```python
from build123d import *

# Parameters (mm, degrees)
BOSS_EXTRUDE1_DEPTH     = 100
BOSS_EXTRUDE2_DEPTH     = 100
CUT_EXTRUDE1_DEPTH      = 10
CHAMFER1_SIZE           = 5.5
CHAMFER2_SIZE           = 4
SKETCH8_R               = 2
BOSS_EXTRUDE3_DEPTH     = 9.3
CUT_EXTRUDE3_DEPTH      = 125.214315536
CUT_EXTRUDE3_DEPTH_BACK = 10
SKETCH9_W               = 11
SKETCH9_H               = 9.3
CHAMFER3_SIZE           = 4
CHAMFER4_SIZE           = 3
CHAMFER5_SIZE           = 3
SKETCH10_W              = 5
SKETCH10_H              = 10
CUT_EXTRUDE4_DEPTH      = 94
CHAMFER7_SIZE           = 1
CHAMFER8_SIZE           = 1
SKETCH11_R              = 2.05
CUT_EXTRUDE5_DEPTH      = 10
CHAMFER9_SIZE           = 0.5
SKETCH12_R              = 2
CUT_EXTRUDE6_DEPTH      = 30
BOSS_EXTRUDE6_START     = -2
BOSS_EXTRUDE6_DEPTH     = 10
SKETCH17_R              = 2
CUT_EXTRUDE7_DEPTH      = 17.1
SKETCH19_W              = 50
SKETCH19_H              = 7
CUT_EXTRUDE13_DEPTH     = 17.1
SKETCH20_W              = 62.3
SKETCH20_H              = 63.674798271
CUT_EXTRUDE14_DEPTH     = 15
CHAMFER10_SIZE          = 5
CHAMFER11_SIZE          = 2


with BuildPart() as part:
    # Sketch4 → Boss-Extrude1 (new body)
    with BuildSketch(Plane.XY):
        Polygon((-18.358738987, 4.974798271), (-27, 4.974798271), (-27, -6.2), (27, -6.2), (27, 4.974798271), (18.358738987, 4.974798271), (21.346410162, -0.2), (-21.346410162, -0.2), align=None)
    extrude(amount=BOSS_EXTRUDE1_DEPTH)

    # Sketch6 → Boss-Extrude2 (add)
    with BuildSketch(Plane.XY.offset(100)):
        Polygon((-24.15, 4.974798271), (-24.15, 52.474798271), (-5.5, 52.474798271), (-5.5, 57.474798271), (-31.15, 57.474798271), (-31.15, -6.2), (-24.15, -6.2), align=None)
        Polygon((24.15, -6.2), (24.15, 52.474798271), (5.5, 52.474798271), (5.5, 57.474798271), (31.15, 57.474798271), (31.15, -6.2), align=None)
    extrude(amount=-BOSS_EXTRUDE2_DEPTH)

    # Sketch7 → Cut-Extrude1 (cut)
    with BuildSketch(Plane(origin=(31.15, 0, 0), x_dir=(0, 0, -1), z_dir=(1, 0, 0))):
        Polygon((-85, 28.724798271), (-81.5, 25.224798271), (-13.5, 25.224798271), (-10, 28.724798271), (-13.5, 32.224798271), (-81.5, 32.224798271), align=None)
    extrude(amount=-CUT_EXTRUDE1_DEPTH, mode=Mode.SUBTRACT)

    # Chamfer1
    chamfer1_edges = [part.edges().sort_by_distance(p)[0] for p in [
        (-24.15, 52.474798271, 50),
        (-24.15, 4.974798271, 50),
        (24.15, 4.974798271, 50),
        (24.15, 52.474798271, 50),
    ]]
    chamfer(chamfer1_edges, length=CHAMFER1_SIZE)

    # Chamfer2
    chamfer2_edges = [part.edges().sort_by_distance(p)[0] for p in [
        (-5.5, 52.474798271, 50),
        (5.5, 52.474798271, 50),
    ]]
    chamfer(chamfer2_edges, length=CHAMFER2_SIZE)

    # Sketch8 → Boss-Extrude3 (add)
    with BuildSketch(Plane(origin=(0, 57.474798271, 0), x_dir=(1, 0, 0), z_dir=(0, 1, 0))):
        Polygon((-21.8, -70), (13.8, -70), (21.8, -62), (21.8, -14), (13.8, -6), (-21.8, -6), align=None)
        with Locations(Location((9.8, -62, 0), (0, 0, 270))):
            Circle(SKETCH8_R, mode=Mode.SUBTRACT)
        with Locations(Location((11.8, -14, 0), (0, 0, 270))):
            Circle(SKETCH8_R, mode=Mode.SUBTRACT)
        with Locations(Location((-11.8, -14, 0), (0, 0, 270))):
            Circle(SKETCH8_R, mode=Mode.SUBTRACT)
        with Locations(Location((-9.8, -62, 0), (0, 0, 270))):
            Circle(SKETCH8_R, mode=Mode.SUBTRACT)
    extrude(amount=BOSS_EXTRUDE3_DEPTH)

    # Sketch9 → Cut-Extrude3 (cut, two sides: drawn at the far end of the back side and taken through both)
    with BuildSketch(Plane.XY.offset(-CUT_EXTRUDE3_DEPTH_BACK)):
        with Locations((0, 62.124798271)):
            Rectangle(SKETCH9_W, SKETCH9_H)
    extrude(amount=CUT_EXTRUDE3_DEPTH + CUT_EXTRUDE3_DEPTH_BACK, mode=Mode.SUBTRACT)

    # Chamfer3
    chamfer3_edges = [part.edges().sort_by_distance(p)[0] for p in [
        (-31.15, -6.2, 50),
        (-31.15, 57.474798271, 50),
        (31.15, -6.2, 50),
        (31.15, 57.474798271, 50),
    ]]
    chamfer(chamfer3_edges, length=CHAMFER3_SIZE)

    # Chamfer4
    chamfer4_edges = [part.edges().sort_by_distance(p)[0] for p in [
        (9.65, 57.474798271, 70),
        (-21.8, 57.474798271, 38),
        (-13.65, 57.474798271, 70),
        (17.8, 57.474798271, 66),
        (21.8, 57.474798271, 38),
        (17.8, 57.474798271, 10),
        (9.65, 57.474798271, 6),
        (-13.65, 57.474798271, 6),
    ]]
    chamfer(chamfer4_edges, length=CHAMFER4_SIZE)

    # Chamfer5
    # the kernel refuses this chamfer: 3 mm, written as the material it adds along each edge
    with BuildSketch(Plane(origin=(31.15, 25.224798271, 81.5), x_dir=(0, -0.014760203742521738, -0.9998910622590239), z_dir=(-1, 0, 0)), Plane(origin=(31.15, 32.224798271, 81.5), x_dir=(0, -0.6965927104131427, 0.7174667907292097), z_dir=(-1, 0, 0))) as chamfer5_piece_1:
        Polygon((CHAMFER5_SIZE * 0.999891062259, -CHAMFER5_SIZE * 0.0147602037425), (-CHAMFER5_SIZE * 0.717466790729, -CHAMFER5_SIZE * 0.696592710413), (0, 0), align=None)
    extrude(amount=7)
    with BuildSketch(Plane(origin=(31.15, 28.724798271, 85), x_dir=(0, 0.7262819568766863, -0.687396915264661), z_dir=(-1, 0, 0))) as chamfer5_piece_2:
        Polygon((CHAMFER5_SIZE * 0.999621916911, CHAMFER5_SIZE * 0.0274958766106), (-CHAMFER5_SIZE * 0.0274958766106, CHAMFER5_SIZE * 0.999621916911), (0, 0), align=None)
    extrude(amount=7)

    # Sketch10 → Cut-Extrude4 (cut)
    with BuildSketch(Plane.XY.offset(100)):
        with Locations((-24.15, 28.724798271)):
            Rectangle(SKETCH10_W, SKETCH10_H)
    extrude(amount=-CUT_EXTRUDE4_DEPTH, mode=Mode.SUBTRACT)

    # Chamfer7
    chamfer7_edges = [part.edges().sort_by_distance(p)[0] for p in [
        (-24.15, 28.724798271, 6),
    ]]
    chamfer(chamfer7_edges, length=CHAMFER7_SIZE)

    # Chamfer8
    chamfer8_edges = [part.edges().sort_by_distance(p)[0] for p in [
        (-24.15, 23.724798271, 52.5),
        (-24.15, 33.724798271, 52.5),
    ]]
    chamfer(chamfer8_edges, length=CHAMFER8_SIZE)

    # Sketch11 → Cut-Extrude5 (cut)
    with BuildSketch(Plane(origin=(0, 66.774798271, 0), x_dir=(1, 0, 0), z_dir=(0, 1, 0))):
        with Locations(Location((-11.8, -14, 0), (0, 0, 270))):
            Circle(SKETCH11_R)
        with Locations(Location((11.8, -14, 0), (0, 0, 270))):
            Circle(SKETCH11_R)
        with Locations(Location((-9.8, -62, 0), (0, 0, 270))):
            Circle(SKETCH11_R)
        with Locations(Location((9.8, -62, 0), (0, 0, 270))):
            Circle(SKETCH11_R)
    extrude(amount=-CUT_EXTRUDE5_DEPTH, mode=Mode.SUBTRACT)

    # Chamfer9
    chamfer9_edges = [part.edges().sort_by_distance(p)[0] for p in [
        (11.8, 66.774798271, 11.95),
        (-9.8, 66.774798271, 59.95),
        (9.8, 66.774798271, 59.95),
        (-11.8, 66.774798271, 11.95),
    ]]
    chamfer(chamfer9_edges, length=CHAMFER9_SIZE)

    # Sketch12 → Cut-Extrude6 (cut)
    with BuildSketch(Plane.XY.offset(100)):
        with Locations((-25, 52.724798271)):
            Circle(SKETCH12_R)
        with Locations((25, 52.724798271)):
            Circle(SKETCH12_R)
        with Locations((-25, 2.724798271)):
            Circle(SKETCH12_R)
        with Locations((25, 2.724798271)):
            Circle(SKETCH12_R)
    extrude(amount=-CUT_EXTRUDE6_DEPTH, mode=Mode.SUBTRACT)

    # Sketch16 → Boss-Extrude6 (add)
    with BuildSketch(Plane(origin=(0, 0, 48), x_dir=(-1, 0, 0), z_dir=(0, 0, -1)).offset(BOSS_EXTRUDE6_START)):
        Polygon((-22, -0.675201729), (22, -0.675201729), (22, -9.250201729), (14.5, -17.825201729), (-14.5, -17.825201729), (-22, -9.250201729), align=None)
        Polygon((-29, 50.324798271), (-37.575, 50.324798271), (-46.15, 42.824798271), (-46.15, 13.824798271), (-37.575, 6.324798271), (-29, 6.324798271), align=None)
        Polygon((37.575, 6.324798271), (29, 6.324798271), (29, 50.324798271), (37.575, 50.324798271), (46.15, 42.824798271), (46.15, 13.824798271), align=None)
    extrude(amount=BOSS_EXTRUDE6_DEPTH)

    # Sketch17 → Cut-Extrude7 (cut)
    with BuildSketch(Plane.XY.offset(50)):
        with Locations((-40.15, 36.724798271)):
            Circle(SKETCH17_R)
        with Locations((-40.15, 20.724798271)):
            Circle(SKETCH17_R)
        with Locations(Location((40.15, 20.724798271, 0), (0, 0, 180))):
            Circle(SKETCH17_R)
        with Locations(Location((40.15, 36.724798271, 0), (0, 0, 180))):
            Circle(SKETCH17_R)
        with Locations((-8, -11.825201729)):
            Circle(SKETCH17_R)
        with Locations((8, -11.825201729)):
            Circle(SKETCH17_R)
    extrude(amount=-CUT_EXTRUDE7_DEPTH, mode=Mode.SUBTRACT)

    # Sketch19 → Cut-Extrude13 (cut)
    with BuildSketch(Plane(origin=(0, 0, 40), x_dir=(-1, 0, 0), z_dir=(0, 0, -1))):
        with Locations((-49.15, 28.724798271)):
            Rectangle(SKETCH19_W, SKETCH19_H)
    extrude(amount=-CUT_EXTRUDE13_DEPTH, mode=Mode.SUBTRACT)

    # Sketch20 → Cut-Extrude14 (cut)
    with BuildSketch(Plane.XY.offset(100)):
        with Locations((0, 25.637399136)):
            Rectangle(SKETCH20_W, SKETCH20_H)
    extrude(amount=-CUT_EXTRUDE14_DEPTH, mode=Mode.SUBTRACT)

    # Chamfer10
    chamfer10_edges = [part.edges().sort_by_distance(p)[0] for p in [
        (-31.15, 28.324798271, 40),
        (31.15, 41.274798271, 40),
        (31.15, 15.774798271, 40),
    ]]
    chamfer(chamfer10_edges, length=CHAMFER10_SIZE)

    # Chamfer11
    chamfer11_edges = [part.edges().sort_by_distance(p)[0] for p in [
        (0, -6.2, 40),
    ]]
    chamfer(chamfer11_edges, length=CHAMFER11_SIZE)


solid = part.part
```
The listing builds one solid part. Answer for the finished solid, in the listing's coordinates (mm). A direction names the side the tool comes from. Round coordinates to 2 decimals unless told otherwise and drop trailing zeros. Write each loop counter-clockwise with the first axis right and the second up, starting at its lowest first coordinate (ties: lowest second). Pieces come first, ordered by that corner, then holes. Notation, with made-up numbers: (39.5, 11) -> (75.5, 11) arc R15 ccw to (75.5, 38) -> close; hole circle Ø6 at (-17, 62). An arc over 180 degrees is marked (long way). Answer as a JSON object with one key per item and string values. Group by question number.
Q1. Each of these flat-tipped pins is pushed along its axis until it touches: pin 1 Ø2 at (x, z) = (17.5, 23.5) entering from -Y; pin 2 Ø2.5 at (y, z) = (-8, 45) entering from -X; pin 3 Ø2 at (x, z) = (-28, 43) entering from +Y. Where does it stop, or does it pass through?
Q2. Which of the six approach directions +Z, -Z, +X, -X, +Y, -Y give full straight-line access (tool end or side, diameter ignored) to faces 4 (the face through (25, 53, 70)), 5 (the face through (-22, -8, 44)), 6 (the face through (14, 52.475, 43)), 7 (the face through (10, 56.775, 62))?
Q3. Straight lines are drawn through the part: line 1 along X through (y, z) = (61, 62); line 2 along Y through (x, z) = (-24.5, 76); line 3 along Y through (x, z) = (-25, 80). For each, find the intervals that lie inside material, in ascending order.
Q4. Section A-A (x = -40.15) is taken. Write down the section's boundary in (y, z).
Q5. Section B-B (x = -2) is taken. Write down the section's boundary in (y, z).
Q6. Determine the mould class of faces 1 (the face through (0, -2, 85)), 2 (the face through (-26.65, 29, 46)), 3 (the face through (-15.015, 58.996, 4.521)) for opening direction Y: pulls with the +Y half, pulls with the -Y half, needs draft (parallel to the pull), parting line crosses it, or undercut.
Check values:
{
 "1": {"pin 1": "y = -6.2", "pin 2": "x = -22", "pin 3": "y = 57.47"},
 "2": {"face 4": "+Z", "face 5": "+Z, -Z, -X, -Y", "face 6": "+Z, -Z", "face 7": "+Y"},
 "3": {"line 1": "-21.8 to -11.85, -7.75 to -5.5, 5.5 to 7.75, 11.85 to 21.8", "line 2": "-6.2 to 0.79, 4.66 to 23.07, 34.37 to 50.79, 54.66 to 57.47", "line 3": "-6.2 to 0.72, 4.72 to 23.57, 33.87 to 50.72, 54.72 to 57.47"},
 "4": {"outline": "(8.58, 40) -> (18.72, 40) -> (18.72, 50) -> (8.58, 50) -> close; (22.72, 40) -> (34.72, 40) -> (34.72, 50) -> (22.72, 50) -> close; (38.72, 40) -> (48.07, 40) -> (48.07, 50) -> (38.72, 50) -> close"},
 "5": {"outline": "(-17.83, 40) -> (-8.2, 40) -> (-6.2, 38) -> (-6.2, 0) -> (-0.2, 0) -> (-0.2, 85) -> (-6.2, 85) -> (-6.2, 50) -> (-17.83, 50) -> close"},
 "6": {"face 1": "needs draft", "face 2": "undercut", "face 3": "pulls with the +Y half"}
}
